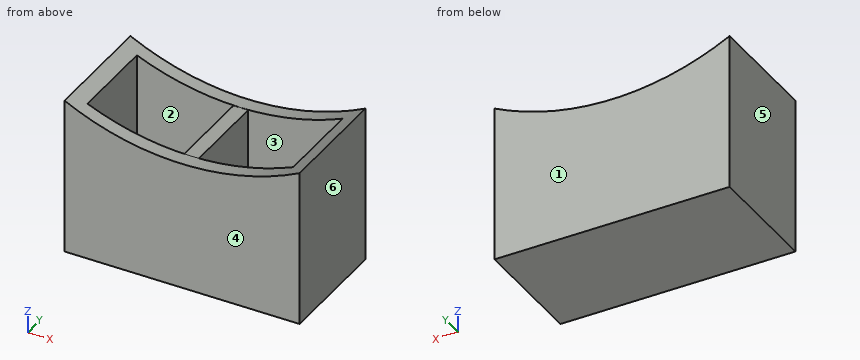
```python
from build123d import *

# Parameters (mm, degrees)
BOSS_EXTRUDE2_DEPTH = 25.4
CUT_EXTRUDE1_START  = -3.175
SKETCH3_W           = 44.45
SKETCH3_H           = 19.05
CUT_EXTRUDE1_DEPTH  = 50.624586707
SKETCH4_W           = 3.175
SKETCH4_H           = 25.4
BOSS_EXTRUDE3_DEPTH = 27.94


with BuildPart() as part:
    # Sketch1 → Boss-Extrude2 (new body)
    with BuildSketch(Plane(origin=(0, 0, 0), x_dir=(1, 0, 0), z_dir=(0, 1, 0))):
        with BuildLine():
            Line((31.360925226, 34.045979578), (-19.439074774, 34.045979578))
            Line((-19.439074774, 34.045979578), (-19.439074774, 0))
            Line((-19.439074774, 0), (-19.437550774, 0))
            ThreePointArc((-19.437550774, 0), (5.961687226, 6.105979578), (31.360925226, 0))
            Line((31.360925226, 0), (31.360925226, 34.045979578))
        make_face()
    extrude(amount=BOSS_EXTRUDE2_DEPTH)

    # Sketch3 → Cut-Extrude1 (cut, through all)
    with BuildSketch(Plane(origin=(0, 0, -34.045979578), x_dir=(-1, 0, 0), z_dir=(0, 0, -1)).offset(CUT_EXTRUDE1_START)):
        with Locations((-5.962449226, 12.7)):
            Rectangle(SKETCH3_W, SKETCH3_H)
    extrude(amount=-CUT_EXTRUDE1_DEPTH, mode=Mode.SUBTRACT)

    # Sketch4 → Boss-Extrude3 (add)
    with BuildSketch(Plane(origin=(0, 0, -34.045979578), x_dir=(-1, 0, 0), z_dir=(0, 0, -1))):
        with Locations((-6.214925226, 12.7)):
            Rectangle(SKETCH4_W, SKETCH4_H)
    extrude(amount=-BOSS_EXTRUDE3_DEPTH)


solid = part.part
```
Input: part model. Units: mm. Frame: model coordinates. Face numbers are marked on the shaded views. A direction names the side the tool comes from. Coordinates: 2 decimals unless noted, no trailing zeros. Loops run counter-clockwise (first coordinate to the right, second up) from the corner with the lowest first, then second, coordinate; pieces in that order, holes last. Notation, with made-up numbers: (11.5, 13.25) - (34.5, 13.25) arc R22 cw to (34.5, 40.25) - close; hole circle Ø9 at (-24.5, 40). An arc over 180 degrees is marked (long way). Answer in a Markdown table with one row per item.
(1) Set-up query: the marked faces 1 and 2. Return all of +Z, -Z, +X, -X, +Y, -Y with unobstructed straight access to the full face (end or side cutting, diameter ignored); none if empty.
Model answer:
| item | result |
|---|---|
| face 1 | +Z, -Z, +X, -X, +Y |
| face 2 | +Z |
(2) Pin query (flat end, axial travel): P1, Ø9.5, axis at x = 17.5, y = 9.5, coming from the +Z side; P2, Ø1, axis at x = 6, y = 14, coming from the +Z side. Return the tip coordinate at first contact, or that it passes through.
Model answer:
| item | result |
|---|---|
| P1 | stops at z = -30.87 |
| P2 | stops at z = -6.11 |
(3) Cut plane D-D on x = 11.5. Output: boundary loops of the cut face in (y, z) (3 decimals), plus the area to 3 significant figures.
Model answer:
| item | result |
|---|---|
| outline | (0, -34.046) - (25.4, -34.046) - (25.4, -5.831) - (22.225, -5.831) - (22.225, -30.871) - (3.175, -30.871) - (3.175, -5.831) - (0, -5.831) - close |
| area | 240 mm² |
(4) Mould query, pull axis X, two halves, no side actions, for the marked faces 3, 4, 5 and 6. Classes: pulls with the +X half, pulls with the -X half, needs draft (parallel to the pull), parting line crosses it, or undercut.
Model answer:
| item | result |
|---|---|
| face 3 | undercut |
| face 4 | needs draft |
| face 5 | pulls with the -X half |
| face 6 | pulls with the +X half |
(5) Cut plane A-A on z = -8. Output: boundary loops of the cut face in (x, y) (3 decimals), plus the area to 3 significant figures.
Model answer:
| item | result |
|---|---|
| outline | (-19.439, 0) - (31.361, 0) - (31.361, 25.4) - (-19.439, 25.4) - close; hole (-16.263, 3.175) - (4.627, 3.175) - (4.627, 22.225) - (-16.263, 22.225) - close; hole (7.802, 3.175) - (28.187, 3.175) - (28.187, 22.225) - (7.802, 22.225) - close |
| area | 504 mm² |
(6) Cut plane B-B on z = -4. Output: boundary loops of the cut face in (x, y) (3 decimals), plus the area to 3 significant figures.
Model answer:
| item | result |
|---|---|
| outline | (-19.439, 0) - (-9.235, 0) - (-9.235, 3.175) - (-16.263, 3.175) - (-16.263, 22.225) - (-9.235, 22.225) - (-9.235, 25.4) - (-19.439, 25.4) - close; (21.158, 0) - (31.361, 0) - (31.361, 25.4) - (21.158, 25.4) - (21.158, 22.225) - (28.187, 22.225) - (28.187, 3.175) - (21.158, 3.175) - close |
| area | 251 mm² |
(7) Material intervals for L1, parallel to X at y = 4.5, z = -27; L2, parallel to Y at x = 0, z = -10.5 (3 decimals); L3, parallel to Z at x = 20.5, y = 14.5, sorted ascending. Write a range as from..to.
Model answer:
| item | result |
|---|---|
| L1 | x = -19.44..-16.26, 4.63..7.8, 28.19..31.36 |
| L2 | y = 0..3.175, 22.225..25.4 |
| L3 | z = -34.05..-30.87 |
